from build123d import *

# Parameters (mm, degrees)
CROQUIS1_W                 = 42
CROQUIS1_H                 = 5
SALIENTE_EXTRUIR1_DEPTH    = 30
CORTAR_EXTRUIR1_DEPTH      = 15
CORTAR_EXTRUIR1_DEPTH_BACK = 21
CROQUIS2_R                 = 1.6
CORTAR_EXTRUIR2_DEPTH      = 2.8
CROQUIS4_W                 = 20
CROQUIS4_H                 = 7
SALIENTE_EXTRUIR2_DEPTH    = 20
FILLET1_R                  = 9
CUT_EXTRUDE1_DEPTH         = 15
CUT_EXTRUDE1_DEPTH_BACK    = 32
SKETCH1_R                  = 2
FILLET2_R                  = 10


with BuildPart() as part:
    # Croquis1 → Saliente-Extruir1 (new body)
    with BuildSketch(Plane.XY):
        with Locations((0, 2.5)):
            Rectangle(CROQUIS1_W, CROQUIS1_H)
    extrude(amount=SALIENTE_EXTRUIR1_DEPTH)

    # Croquis2 → Cortar-Extruir1 (cut, two sides: drawn at the far end of the back side and taken through both)
    with BuildSketch(Plane(origin=(0, 5, 0), x_dir=(1, 0, 0), z_dir=(0, 1, 0)).offset(-CORTAR_EXTRUIR1_DEPTH_BACK)):
        with Locations((-17, -15)):
            Circle(CROQUIS2_R)
        with Locations((17, -15)):
            Circle(CROQUIS2_R)
    extrude(amount=CORTAR_EXTRUIR1_DEPTH + CORTAR_EXTRUIR1_DEPTH_BACK, mode=Mode.SUBTRACT)

    # Croquis3 → Cortar-Extruir2 (cut)
    with BuildSketch(Plane(origin=(0, 5, 0), x_dir=(1, 0, 0), z_dir=(0, 1, 0))):
        Polygon((15.383419246, -17.8), (13.766838493, -15), (15.383419246, -12.2), (18.616580754, -12.2), (20.233161507, -15), (18.616580754, -17.8), align=None)
        Polygon((-13.766838493, -15), (-15.383419246, -12.2), (-18.616580754, -12.2), (-20.233161507, -15), (-18.616580754, -17.8), (-15.383419246, -17.8), align=None)
    extrude(amount=-CORTAR_EXTRUIR2_DEPTH, mode=Mode.SUBTRACT)

    # Croquis4 → Saliente-Extruir2 (add)
    with BuildSketch(Plane(origin=(0, 5, 0), x_dir=(1, 0, 0), z_dir=(0, 1, 0))):
        with Locations((-0.205428596, -22)):
            Rectangle(CROQUIS4_W, CROQUIS4_H)
        with Locations((-0.205428596, -8)):
            Rectangle(CROQUIS4_W, CROQUIS4_H)
    extrude(amount=SALIENTE_EXTRUIR2_DEPTH)

    # Fillet1
    fillet1_edges = [part.edges().sort_by_distance(p)[0] for p in [
        (-10.205428596, 25, 22),
        (9.794571404, 25, 22),
        (-10.205428596, 25, 8),
        (9.794571404, 25, 8),
    ]]
    fillet(fillet1_edges, radius=FILLET1_R)

    # Sketch1 → Cut-Extrude1 (cut, two sides: drawn at the far end of the back side and taken through both)
    with BuildSketch(Plane.XY.offset(25.5).offset(-CUT_EXTRUDE1_DEPTH_BACK)):
        with Locations(Location((0, 16, 0), (0, 0, 180))):
            Circle(SKETCH1_R)
    extrude(amount=CUT_EXTRUDE1_DEPTH + CUT_EXTRUDE1_DEPTH_BACK, mode=Mode.SUBTRACT)

    # Fillet2
    fillet2_edges = [part.edges().sort_by_distance(p)[0] for p in [
        (-10.205428596, 5, 22),
        (9.794571404, 5, 22),
        (-10.205428596, 5, 8),
        (9.794571404, 5, 8),
    ]]
    fillet(fillet2_edges, radius=FILLET2_R)


solid = part.part
Verification items for the finished model (mm, model axes). A direction names the side the tool comes from. Coordinates: 2 decimals unless noted, no trailing zeros. Loops run counter-clockwise (first coordinate to the right, second up) from the corner with the lowest first, then second, coordinate; pieces in that order, holes last. Notation, with made-up numbers: (2, -8) -> (37, -8) arc R8 ccw to (37, -2) -> close; hole circle Ø5 at (81.25, 50). An arc over 180 degrees is marked (long way). Answer as a JSON object with one key per item and string values. Group by question number.
Item 1: Mould release check, pull along X, two halves, no side actions. Record for faces 1 (the flat face through (9.795, 15.5, 8)), 2 (the flat face through (-21, 2, 15)), 3 (the flat face through (-15.6, 2.2, 13.7)): +X half, -X half, draft (parallel to the pull), parting line (faces both ways), or undercut.
Item 2: Sectioned sample at B-B on z = 19. Record the boundary of the cut face in (x, y).
Item 3: Scan lines: probe 1 along Z at (x, y) = (4.5, 22.25); probe 2 along Y at (x, z) = (19.5, 20.75); probe 3 along Z at (x, y) = (17, 1.5). Record each from-to range of solid material in increasing order.
Item 4: Sectioned sample at A-A on x = 0. Record the boundary of the cut face in (y, z), plus the area to 3 significant figures.
Item 5: Depth check by flat-ended pin: pin 1 (1.7 mm diameter, centred on x = 18.5, z = 13.5, fed in from +Y); pin 2 (8 mm diameter, centred on y = 12.5, z = 12.5, fed in from -X); pin 3 (0.5 mm diameter, centred on y = 15.5, z = 23, fed in from +X). Enter the tip coordinate at first touch or a pass-through.
Item 6: Sectioned sample at C-C on y = 9.25. Record the boundary of the cut face in (x, z), plus the area to 3 significant figures.
Item 7: Sectioned sample at D-D on x = 18. Record the boundary of the cut face in (y, z), plus the area to 3 significant figures.
Item 8: Tool access check on faces 4 (the flat face through (-10.205, 15.5, 8)), 5 (the flat face through (0, 13, 18.5)), 6 (the flat face through (-19.414, 3.62, 13.58)), 7 (the flat face through (9.795, 15.5, 22)). Record the directions out of +Z, -Z, +X, -X, +Y, -Y that give a thin tool (end or side, any length) a straight path to the whole face; none if there is none.
Evaluation:
{
 "1": {"face 1": "+X half", "face 2": "-X half", "face 3": "undercut"},
 "2": {"outline": "(-21, 0) -> (21, 0) -> (21, 5) -> (19.79, 5) arc R10 cw to (9.79, 15) -> (9.79, 16) arc R9 ccw to (0.79, 25) -> (-1.21, 25) arc R9 ccw to (-10.21, 16) -> (-10.21, 15) arc R10 cw to (-20.21, 5) -> (-21, 5) -> close; hole circle Ø4 at (0, 16)"},
 "3": {"probe 1": "z = 4.5 to 11.5, 18.5 to 25.5", "probe 2": "y = 0 to 5", "probe 3": "z = 0 to 13.4, 16.6 to 30"},
 "4": {"outline": "(0, 0) -> (5, 0) -> (5, 4.5) -> (14, 4.5) -> (14, 11.5) -> (5, 11.5) -> (5, 18.5) -> (14, 18.5) -> (14, 25.5) -> (5, 25.5) -> (5, 30) -> (0, 30) -> close; (18, 4.5) -> (25, 4.5) -> (25, 11.5) -> (18, 11.5) -> close; (18, 18.5) -> (25, 18.5) -> (25, 25.5) -> (18, 25.5) -> close", "area": "374 mm²"},
 "5": {"pin 1": "stops at y = 5", "pin 2": "stops at x = -12.5", "pin 3": "stops at x = 9.79"},
 "6": {"outline": "(-12.02, 4.5) -> (11.61, 4.5) -> (11.61, 11.5) -> (-12.02, 11.5) -> close; (-12.02, 18.5) -> (11.61, 18.5) -> (11.61, 25.5) -> (-12.02, 25.5) -> close", "area": "331 mm²"},
 "7": {"outline": "(0, 0) -> (5, 0) -> (5, 4.5) -> (5.16, 4.5) -> (5.16, 11.5) -> (5, 11.5) -> (5, 12.2) -> (2.2, 12.2) -> (2.2, 13.75) -> (0, 13.75) -> close; (0, 16.25) -> (2.2, 16.25) -> (2.2, 17.8) -> (5, 17.8) -> (5, 18.5) -> (5.16, 18.5) -> (5.16, 25.5) -> (5, 25.5) -> (5, 30) -> (0, 30) -> close", "area": "131 mm²"},
 "8": {"face 4": "+Z, -Z, -X, +Y", "face 5": "+X, -X, +Y", "face 6": "+Y", "face 7": "+Z, -Z, +X, +Y"}
}
